Geometry check sheet. Reference: the model listing, model coordinates, mm. A direction names the side the tool comes from. Coordinates: 2 decimals unless noted, no trailing zeros. Write each loop counter-clockwise with the first axis right and the second up, starting at its lowest first coordinate (ties: lowest second). Pieces come first, ordered by that corner, then holes. Notation, with made-up numbers: (-23.5, 50.5) -> (6.5, 50.5) arc R29 ccw to (6.5, 85.5) -> close; hole circle Ø8 at (57, 55.25). An arc over 180 degrees is marked (long way). Answer in a Markdown table with one row per item. Add a question column.
Q1. Section check A-A, the plane z = -7.5. Record the boundary of the cut face in (x, y), and give its area (3 significant figures).
Q2. Tool access check on faces 1 (the face through (10, 17, 0)), 2 (the face through (-18, 0, -10)), 3 (the face through (10, 0, 18)). Record the directions out of +Z, -Z, +X, -X, +Y, -Y that give a thin tool (end or side, any length) a straight path to the whole face; none if there is none.
Q3. Thickness scan on line 1 (Z direction, x = -21.5, y = 6). Record the ranges inside material, lowest first.
Q4. Release check for a two-part mould opening along Y. For faces 4 (the face through (-10, 17, 0)), 5 (the face through (18, 10, 0)), 6 (the face through (0, 25, 11)) record: pulls with the +Y half, pulls with the -Y half, needs draft (parallel to the pull), parting line crosses it, or undercut.
Q5. Section check B-B, the plane x = 11. Record the boundary of the cut face in (y, z).
```python
from build123d import *

# Parameters (mm, degrees)
F0_W      = 50
F0_H      = 50
F1_DEPTH  = 25
F2_W      = 20
F2_H      = 20
F3_DEPTH  = 50
F4_W      = 20
F4_H      = 20
F5_DEPTH  = 15
F6_W      = 20
F6_H      = 20
F7_DEPTH  = 15
F8_W      = 20
F8_H      = 20
F9_DEPTH  = 15
F10_W     = 20
F10_H     = 20
F11_DEPTH = 15


with BuildPart() as f1:
    # F0 (on Front) → F1 (new body, symmetric)
    with BuildSketch(Plane.XZ):
        Rectangle(F0_W, F0_H)
    extrude(amount=F1_DEPTH, both=True)

    # F2 (on face) → F3 (cut, through all)
    with BuildSketch(Plane.XZ.offset(25)):
        Rectangle(F2_W, F2_H)
    extrude(amount=-F3_DEPTH, mode=Mode.SUBTRACT)

    # F4 (on face) → F5 (cut, through all)
    with BuildSketch(Plane(origin=(-25, 0, 0), x_dir=(0, -1, 0), z_dir=(-1, 0, 0))):
        Rectangle(F4_W, F4_H)
    extrude(amount=-F5_DEPTH, mode=Mode.SUBTRACT)

    # F6 (on face) → F7 (cut, through all)
    with BuildSketch(Plane.YZ.offset(25)):
        Rectangle(F6_W, F6_H)
    extrude(amount=-F7_DEPTH, mode=Mode.SUBTRACT)

    # F8 (on face) → F9 (cut, through all)
    with BuildSketch(Plane.XY.offset(25)):
        Rectangle(F8_W, F8_H)
    extrude(amount=-F9_DEPTH, mode=Mode.SUBTRACT)

    # F10 (on face) → F11 (cut, through all)
    with BuildSketch(Plane(origin=(0, 0, -25), x_dir=(1, 0, 0), z_dir=(0, 0, -1))):
        Rectangle(F10_W, F10_H)
    extrude(amount=-F11_DEPTH, mode=Mode.SUBTRACT)


solid = f1.part
```
Calculated:
| question | item | result |
|---|---|---|
| 1 | outline | (-25, -25) -> (-10, -25) -> (-10, -10) -> (-25, -10) -> close; (-25, 10) -> (-10, 10) -> (-10, 25) -> (-25, 25) -> close; (10, -25) -> (25, -25) -> (25, -10) -> (10, -10) -> close; (10, 10) -> (25, 10) -> (25, 25) -> (10, 25) -> close |
| 1 | area | 900 mm² |
| 2 | face 1 | +Y, -Y |
| 2 | face 2 | +X, -X |
| 2 | face 3 | +Z, -Z |
| 3 | line 1 | z = -25 to -10, 10 to 25 |
| 4 | face 4 | needs draft |
| 4 | face 5 | undercut |
| 4 | face 6 | pulls with the +Y half |
| 5 | outline | (-25, -25) -> (25, -25) -> (25, 25) -> (-25, 25) -> close; hole (-10, -10) -> (10, -10) -> (10, 10) -> (-10, 10) -> close |
